Work out the finished part from the listing and answer in its coordinate system (mm). Face numbers are marked on the shaded views. A direction names the side the tool comes from. Coordinates: 2 decimals unless noted, no trailing zeros. Order: outer loops, then holes, each group sorted by start corner. A loop starts at its lowest first (then second) coordinate and runs counter-clockwise, first axis right, second up. Notation, with made-up numbers: M 86,-36 L 135,-36 A7 ccw 135,-26 Z; hole C 83,-7 d9. An arc over 180 degrees is marked long. Use a Markdown table: item, result. Add a question column.
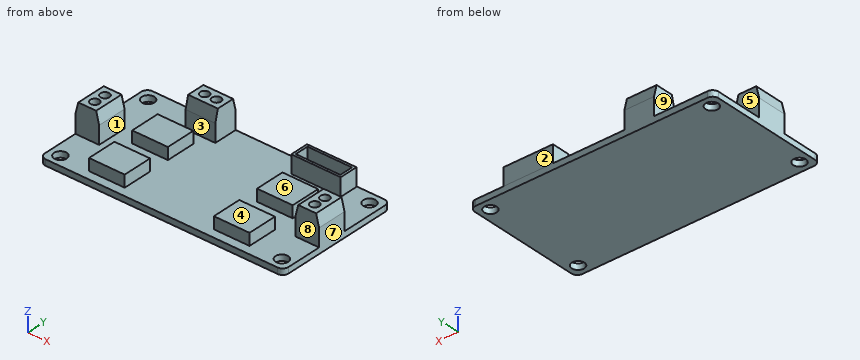
from build123d import *

# Parameters (mm, degrees)
EXTRUDE_1_DEPTH          = 2
SKETCH_2_R               = 2.112337694
CUT_EXTRUDE_1_DEPTH      = 2
MIRROR_2_COPY_1_SKETCH_R = 2.112337694
MIRROR_2_COPY_1_DEPTH    = 2
SKETCH_3_W               = 8
SKETCH_3_H               = 10
EXTRUDE_2_DEPTH          = 10
CUT_EXTRUDE_2_DEPTH      = 10
SKETCH_5_R               = 1.5
CUT_EXTRUDE_3_DEPTH      = 8
SKETCH_6_W               = 10
SKETCH_6_H               = 8
EXTRUDE_3_DEPTH          = 10
CUT_EXTRUDE_4_DEPTH      = 10
SKETCH_8_R               = 1.5
CUT_EXTRUDE_5_DEPTH      = 8
SKETCH_9_W               = 16.6
SKETCH_9_H               = 6.196182774
SKETCH_9_W_2             = 15
SKETCH_9_H_2             = 4.596182774
EXTRUDE_1_2_DEPTH        = 6
SKETCH_10_W              = 12
SKETCH_10_H              = 10
EXTRUDE_4_DEPTH          = 4
SKETCH_12_W              = 12
SKETCH_12_H              = 10
EXTRUDE_5_DEPTH          = 4


with BuildPart() as part:
    # 草图1 → Extrude 1 (new body)
    with BuildSketch(Plane.XY):
        with BuildLine():
            Line((-39, 21), (39, 21))
            ThreePointArc((39, 21), (40.414213562, 20.414213562), (41, 19))
            Line((41, 19), (41, -19))
            ThreePointArc((41, -19), (40.414213562, -20.414213562), (39, -21))
            Line((39, -21), (-39, -21))
            ThreePointArc((-39, -21), (-40.414213562, -20.414213562), (-41, -19))
            Line((-41, -19), (-41, 19))
            ThreePointArc((-41, 19), (-40.414213562, 20.414213562), (-39, 21))
        make_face()
    extrude(amount=EXTRUDE_1_DEPTH)

    # 草图2 → 切除-拉伸1 (cut)
    with BuildSketch(Plane.XY.offset(2)):
        with Locations((-37.25, 17.25)):
            Circle(SKETCH_2_R)
    cut_extrude_1 = extrude(amount=-CUT_EXTRUDE_1_DEPTH, mode=Mode.SUBTRACT)

    # 镜向1: 切除-拉伸1 across plane
    add(cut_extrude_1.mirror(Plane.ZX), mode=Mode.SUBTRACT)

    # 镜向2: 切除-拉伸1 across plane
    add(cut_extrude_1.mirror(Plane(origin=(0, 0, 0), x_dir=(0, 0, 1), z_dir=(1, 0, 0))), mode=Mode.SUBTRACT)

    # 镜向2 copy 1 sketch → 镜向2 copy 1 (cut)
    with BuildSketch(Plane(origin=(0, 0, 2), x_dir=(-1, 0, 0), z_dir=(0, 0, 1))):
        with Locations((-37.25, 17.25)):
            Circle(MIRROR_2_COPY_1_SKETCH_R)
    extrude(amount=-MIRROR_2_COPY_1_DEPTH, mode=Mode.SUBTRACT)

    # 草图3 → 凸台-拉伸2 (add)
    with BuildSketch(Plane.XY.offset(2)):
        with Locations((-37, -2)):
            Rectangle(SKETCH_3_W, SKETCH_3_H)
    extrude_2 = extrude(amount=EXTRUDE_2_DEPTH)

    # 草图4 → 切除-拉伸2 (cut)
    with BuildSketch(Plane.XZ.offset(7)):
        Polygon((-40, 12), (-41, 8), (-41, 12), align=None)
        Polygon((-33, 12), (-34, 12), (-33, 8), align=None)
    cut_extrude_2 = extrude(amount=-CUT_EXTRUDE_2_DEPTH, mode=Mode.SUBTRACT)

    # 草图5 → 切除-拉伸3 (cut)
    with BuildSketch(Plane.XY.offset(12)):
        with Locations((-37, 0)):
            Circle(SKETCH_5_R)
        with Locations((-37, -4)):
            Circle(SKETCH_5_R)
    cut_extrude_3 = extrude(amount=-CUT_EXTRUDE_3_DEPTH, mode=Mode.SUBTRACT)

    # 镜向3: 凸台-拉伸2, 切除-拉伸2, 切除-拉伸3 across plane
    add(extrude_2.mirror(Plane(origin=(0, 0, 0), x_dir=(0, 0, 1), z_dir=(1, 0, 0))))
    add(cut_extrude_2.mirror(Plane(origin=(0, 0, 0), x_dir=(0, 0, 1), z_dir=(1, 0, 0))), mode=Mode.SUBTRACT)
    add(cut_extrude_3.mirror(Plane(origin=(0, 0, 0), x_dir=(0, 0, 1), z_dir=(1, 0, 0))), mode=Mode.SUBTRACT)

    # 草图6 → 凸台-拉伸3 (add)
    with BuildSketch(Plane.XY.offset(2)):
        with Locations((-16, 17)):
            Rectangle(SKETCH_6_W, SKETCH_6_H)
    extrude(amount=EXTRUDE_3_DEPTH)

    # 草图7 → 切除-拉伸4 (cut)
    with BuildSketch(Plane.ZY.offset(21)):
        Polygon((8, 21), (12, 20), (12, 21), align=None)
        Polygon((12, 13), (8, 13), (12, 14), align=None)
    extrude(amount=-CUT_EXTRUDE_4_DEPTH, mode=Mode.SUBTRACT)

    # 草图8 → 切除-拉伸5 (cut)
    with BuildSketch(Plane.XY.offset(12)):
        with Locations((-14, 17)):
            Circle(SKETCH_8_R)
        with Locations((-18, 17)):
            Circle(SKETCH_8_R)
    extrude(amount=-CUT_EXTRUDE_5_DEPTH, mode=Mode.SUBTRACT)

    # 草图9 → Extrude 1 2 (add)
    with BuildSketch(Plane.XY.offset(2)):
        with Locations((21.5, 17.701908613)):
            Rectangle(SKETCH_9_W, SKETCH_9_H)
        with Locations((21.5, 17.701908613)):
            Rectangle(SKETCH_9_W_2, SKETCH_9_H_2, mode=Mode.SUBTRACT)
    extrude(amount=EXTRUDE_1_2_DEPTH)

    # 草图10 → 凸台-拉伸4 (add)
    with BuildSketch(Plane.XY.offset(2)):
        with Locations((-21, 4)):
            Rectangle(SKETCH_10_W, SKETCH_10_H)
    extrude_4 = extrude(amount=EXTRUDE_4_DEPTH)

    # 草图12 → 凸台-拉伸5 (add)
    with BuildSketch(Plane.XY.offset(2)):
        with Locations((-21, -13)):
            Rectangle(SKETCH_12_W, SKETCH_12_H)
    extrude_5 = extrude(amount=EXTRUDE_5_DEPTH)

    # 镜向4: 凸台-拉伸4, 凸台-拉伸5 across plane
    add(extrude_4.mirror(Plane(origin=(0, 0, 0), x_dir=(0, 0, 1), z_dir=(1, 0, 0))))
    add(extrude_5.mirror(Plane(origin=(0, 0, 0), x_dir=(0, 0, 1), z_dir=(1, 0, 0))))


solid = part.part
(1) A cutting plane is placed at B-B on x = -37.25. Write down the section's boundary in (y, z).
(2) Which of the six approach directions +Z, -Z, +X, -X, +Y, -Y give full straight-line access (tool end or side, diameter ignored) to the marked faces 1, 2, 3, 4 and 5?
(3) Given P1, Ø2.5, axis at x = 36.5, z = 7, coming from the +Y side; P2, Ø1.5, axis at x = -36.5, y = 0.5, coming from the +Z side; P3, Ø4.5, axis at x = -24, z = 5, coming from the -Y side, each flat-ended and moving along its own axis, determine where each tip first touches the part or whether it passes through.
(4) A cutting plane is placed at A-A on y = -17.25. Write down the section's boundary in (x, z).
(5) A cutting plane is placed at C-C on y = 0. Write down the section's boundary in (x, z).
(6) Straight lines are drawn through the part: line 1 (Y direction, x = 37.25, z = 1.05); line 2 (X direction, y = 19.5, z = 4.5); line 3 (Y direction, x = 37, z = 6.5). For each, find the intervals that lie inside material, in ascending order.
(7) The mould has two halves that part along X. Classify the marked faces 6, 7, 8 and 9: pulls with the +X half, pulls with the -X half, needs draft (parallel to the pull), parting line crosses it, or undercut.
(8) A cutting plane is placed at D-D on x = -14. Write down the section's boundary in (y, z), plus the area to 3 significant figures.
From the geometry:
| question | item | result |
|---|---|---|
| 1 | outline | M -21,0 L -19.36,0 L -19.36,2 L -21,2 Z; M -15.14,0 L 15.14,0 L 15.14,2 L 3,2 L 3,12 L 1.48,12 L 1.48,4 L -1.48,4 L -1.48,12 L -2.52,12 L -2.52,4 L -5.48,4 L -5.48,12 L -7,12 L -7,2 L -15.14,2 Z; M 19.36,0 L 21,0 L 21,2 L 19.36,2 Z |
| 2 | face 1 | +Z, +Y, -Y |
| 2 | face 2 | +Z, +X, +Y |
| 2 | face 3 | +Z, +X, -X |
| 2 | face 4 | +Z, +X, -X, -Y |
| 2 | face 5 | +Z, -X, +Y |
| 3 | P1 | stops at y = 3 |
| 3 | P2 | stops at z = 4 |
| 3 | P3 | stops at y = -18 |
| 4 | outline | M -41,0 L -39.36,0 L -39.36,2 L -41,2 Z; M -35.14,0 L 35.14,0 L 35.14,2 L 27,2 L 27,6 L 15,6 L 15,2 L -15,2 L -15,6 L -27,6 L -27,2 L -35.14,2 Z; M 39.36,0 L 41,0 L 41,2 L 39.36,2 Z |
| 5 | outline | M -41,0 L 41,0 L 41,8 L 40,12 L 38.5,12 L 38.5,4 L 35.5,4 L 35.5,12 L 34,12 L 33,8 L 33,2 L 27,2 L 27,6 L 15,6 L 15,2 L -15,2 L -15,6 L -27,6 L -27,2 L -33,2 L -33,8 L -34,12 L -35.5,12 L -35.5,4 L -38.5,4 L -38.5,12 L -40,12 L -41,8 Z |
| 6 | line 1 | y = -21 to -19.36, -15.14 to 15.14, 19.36 to 21 |
| 6 | line 2 | x = -21 to -11, 13.2 to 14, 29 to 29.8 |
| 6 | line 3 | y = -7 to -5.5, -2.5 to -1.5, 1.5 to 3 |
| 7 | face 6 | undercut |
| 7 | face 7 | pulls with the +X half |
| 7 | face 8 | needs draft |
| 7 | face 9 | pulls with the -X half |
| 8 | outline | M -21,0 L 21,0 L 21,8 L 20,12 L 18.5,12 L 18.5,4 L 15.5,4 L 15.5,12 L 14,12 L 13,8 L 13,2 L -21,2 Z |
| 8 | area | 136 mm2 |
